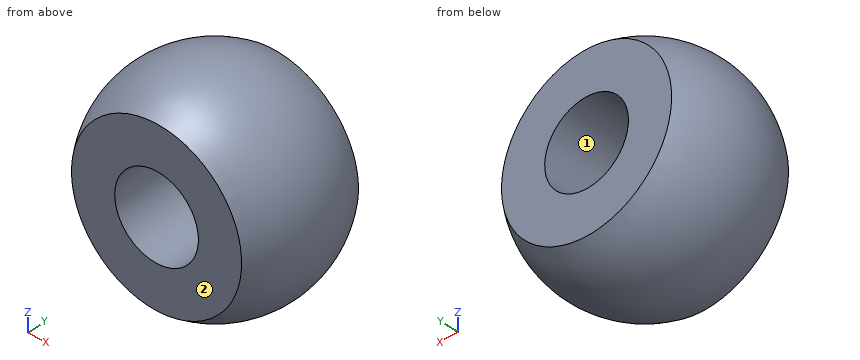
from build123d import *

# Parameters (mm, degrees)
SKETCH1_W           = 65
SKETCH1_H           = 5
BOSS_EXTRUDE1_DEPTH = 5
SKETCH3_R           = 1.65
CUT_EXTRUDE2_DEPTH  = 32.364560159


# Read off the part's stored shape, not the designer's step: Cut-Revolve1
with BuildPart() as part:
    # Sketch1 → Boss-Extrude1 (new, symmetric)
    with BuildSketch(Plane.XY):
        Rectangle(SKETCH1_W, SKETCH1_H)
    extrude(amount=BOSS_EXTRUDE1_DEPTH, both=True)

    # Cut-Revolve1 outline → Cut-Revolve1 (revolve, cut)
    with BuildSketch(Plane.YX):
        with BuildLine():
            Line((5.590169944, -32.5), (5.590169944, 32.5))
            Line((5.590169944, 32.5), (0, 32.5))
            Line((0, 32.5), (0, -22.319988038))
            ThreePointArc((0, -22.319988038), (4.180011962, -26.5), (0, -30.680011962))
            Line((0, -30.680011962), (0, -32.5))
            Line((0, -32.5), (5.590169944, -32.5))
        make_face()
    revolve(axis=Axis((0, 0, 0), (1, 0, 0)), mode=Mode.SUBTRACT)

    # Sketch3 → Cut-Extrude2 (cut, through all)
    with BuildSketch(Plane(origin=(0, 2.5, 0), x_dir=(1, 0, 0), z_dir=(0, 1, 0))):
        with Locations(Location((-26.5, 0, 0), (0, 0, 270))):
            Circle(SKETCH3_R)
    extrude(amount=-CUT_EXTRUDE2_DEPTH, mode=Mode.SUBTRACT)


solid = part.part
The model under review builds one solid part; all positions refer to its coordinate system, in mm. Face numbers are marked on the shaded views. Round coordinates to 2 decimals unless told otherwise and drop trailing zeros. Loops run counter-clockwise (first coordinate to the right, second up) from the corner with the lowest first, then second, coordinate; pieces in that order, holes last. Notation, with made-up numbers: M 13,47 L 68,47 A31 cw 68,73 Z; hole C -7,-0.5 d9. An arc over 180 degrees is marked long. Answer as a JSON object with one key per item and string values.
Item 1: We need section A-A, the plane x = -26.5. State the section outline as (y, z) points.
Check sheet entries:
{"outline": "M -2.5,-3.35 A4.18 ccw 2.5,-3.35 L 2.5,-1.65 L -2.5,-1.65 Z; M -2.5,1.65 L 2.5,1.65 L 2.5,3.35 A4.18 ccw -2.5,3.35 Z"}
Item 2: We need section D-D, the plane x = -23.75. State the section outline as (y, z) points, and give its area (3 significant figures).
Check sheet entries:
{"outline": "M -2.5,-1.91 A3.15 ccw 2.5,-1.91 L 2.5,1.91 A3.15 ccw -2.5,1.91 Z", "area": "27.8 mm2"}
Item 3: We need section B-B, the plane z = 0. State the section outline as (x, y) points, and give its area (3 significant figures).
Check sheet entries:
{"outline": "M -29.85,-2.5 L -28.15,-2.5 L -28.15,2.5 L -29.85,2.5 A4.18 ccw Z; M -24.85,-2.5 L -23.15,-2.5 A4.18 ccw -23.15,2.5 L -24.85,2.5 Z", "area": "22.7 mm2"}
Item 4: Clearance check with flat-ended pins moving along their axes: P1, Ø1.5, axis at y = 0.5, z = 1, coming from the +X side; P2, Ø2.5, axis at x = -26.5, z = 0, coming from the +Y side. State where each tip first meets the part, or that it passes through.
Check sheet entries:
{"P1": "x = -22.34", "P2": "through"}
Item 5: For line 1 along X through (y, z) = (1.75, 0); line 2 along X through (y, z) = (1.25, 0); line 3 along Z through (x, y) = (-26.25, 1.55), list the stretches that pass through material, from the lowest coordinate up.
Check sheet entries:
{"line 1": "-30.3 to -28.15, -24.85 to -22.7", "line 2": "-30.49 to -28.15, -24.85 to -22.51", "line 3": "-3.87 to -1.63, 1.63 to 3.87"}
Item 6: We need section C-C, the plane y = -0.7. State the section outline as (x, z) points.
Check sheet entries:
{"outline": "C -26.5,0 d8.24; hole C -26.5,0 d3.3"}
Item 7: The part is to be moulded in two halves that separate along X. For the marked faces 1 and 2, say which applies: +X half, -X half, draft (parallel to the pull), parting line (faces both ways), or undercut.
Check sheet entries:
{"face 1": "undercut", "face 2": "draft"}
